Study the drawing (mm; zero at the part's minimum x, y, z) and answer. Round coordinates to 2 decimals unless told otherwise and drop trailing zeros. Loops run counter-clockwise (first coordinate to the right, second up) from the corner with the lowest first, then second, coordinate; pieces in that order, holes last. Notation, with made-up numbers: (6.25, 26.5) - (64.25, 26.5) arc R14 cw to (64.25, 33.5) - close; hole circle Ø8 at (-30.5, 8.5). An arc over 180 degrees is marked (long way). One line per item, written item: value.
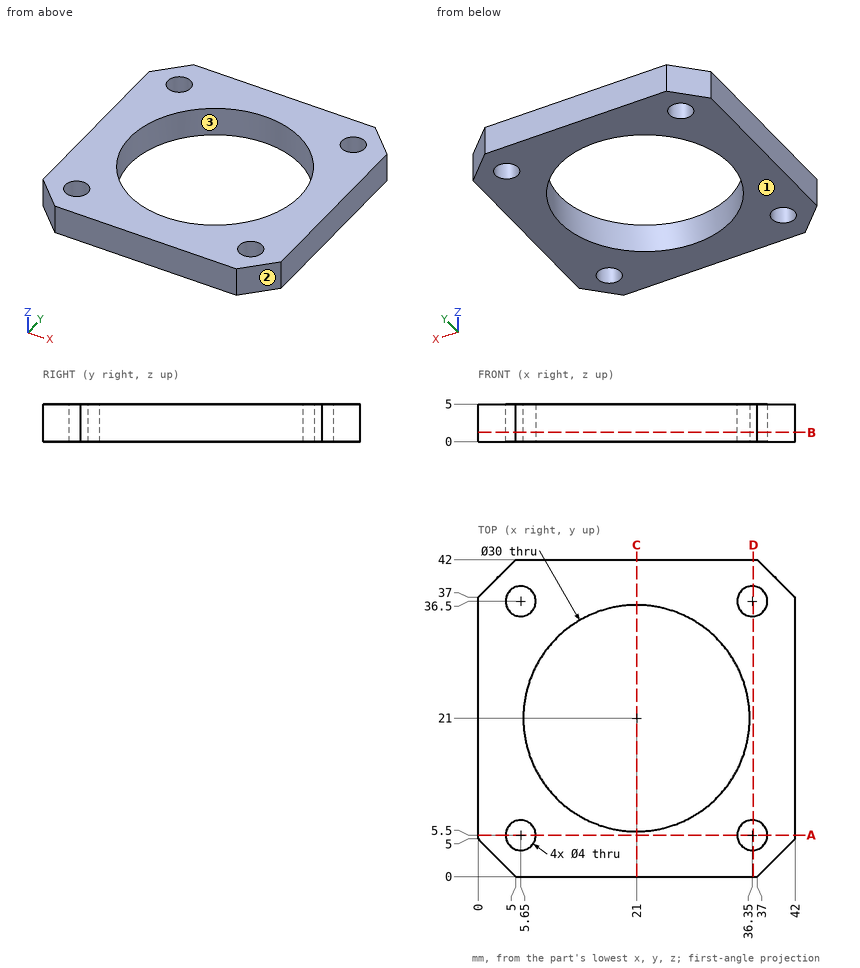
1) A cutting plane is placed at C-C on x = 21. Give the vertices of the cut face in (y, z), and give its area (3 significant figures).
Final values:
outline: (0, 0) - (6, 0) - (6, 5) - (0, 5) - close; (36, 0) - (42, 0) - (42, 5) - (36, 5) - close
area: 60.0 mm2
2) For a pull along Y with two mould halves and no side action, classify the marked faces 1, 2 and 3 as released by +Y, released by -Y, zero draft, split by the parting line, or undercut.
Final values:
face 1: zero draft
face 2: released by -Y
face 3: undercut
3) Consider L1, parallel to Y at x = 36.35, z = 3.5; L2, parallel to Y at x = 21, z = 4.25; L3, parallel to Y at x = 13.5, z = 3.4. Determine where each line is inside the solid, lowest interval first.
Final values:
L1: 0 to 3.5, 7.5 to 34.5, 38.5 to 42
L2: 0 to 6, 36 to 42
L3: 0 to 8.01, 33.99 to 42
4) A cutting plane is placed at A-A on y = 5.5. Give the vertices of the cut face in (x, z), and give its area (3 significant figures).
Final values:
outline: (0, 0) - (3.65, 0) - (3.65, 5) - (0, 5) - close; (7.65, 0) - (34.35, 0) - (34.35, 5) - (7.65, 5) - close; (38.35, 0) - (42, 0) - (42, 5) - (38.35, 5) - close
area: 170 mm2
5) A cutting plane is placed at D-D on x = 36.5. Give the vertices of the cut face in (y, z).
Final values:
outline: (0, 0) - (3.51, 0) - (3.51, 5) - (0, 5) - close; (7.49, 0) - (34.51, 0) - (34.51, 5) - (7.49, 5) - close; (38.49, 0) - (42, 0) - (42, 5) - (38.49, 5) - close
6) A cutting plane is placed at B-B on z = 1.25. Give the vertices of the cut face in (x, y), and give its area (3 significant figures).
Final values:
outline: (0, 5) - (5, 0) - (37, 0) - (42, 5) - (42, 37) - (37, 42) - (5, 42) - (0, 37) - close; hole circle Ø4 at (5.65, 5.5); hole circle Ø4 at (5.65, 36.5); hole circle Ø30 at (21, 21); hole circle Ø4 at (36.35, 5.5); hole circle Ø4 at (36.35, 36.5)
area: 957 mm2
